Source: CAD feature listing. Evaluate the final solid. Frame: model axes, mm. Face numbers are marked on the shaded views. A direction names the side the tool comes from. Give positions to 0.01 mm unless a question says otherwise; leave off trailing zeros. Order: outer loops, then holes, each group sorted by start corner. A loop starts at its lowest first (then second) coordinate and runs counter-clockwise, first axis right, second up.
from build123d import *

# Parameters (mm, degrees)
SKETCH1_R           = 1.5
BOSS_EXTRUDE1_DEPTH = 1.5


with BuildPart() as part:
    # Sketch1 → Boss-Extrude1 (new body, symmetric)
    with BuildSketch(Plane.XY):
        with BuildLine():
            Line((-10.75, 18.625), (10.75, 18.625))
            ThreePointArc((10.75, 18.625), (14.25, 15.125), (10.75, 11.625))
            ThreePointArc((10.75, 11.625), (8.275126266, 10.599873734), (7.25, 8.125))
            Line((7.25, 8.125), (7.25, -8.125))
            ThreePointArc((7.25, -8.125), (8.275126266, -10.599873734), (10.75, -11.625))
            ThreePointArc((10.75, -11.625), (14.25, -15.125), (10.75, -18.625))
            Line((10.75, -18.625), (-10.75, -18.625))
            ThreePointArc((-10.75, -18.625), (-14.25, -15.125), (-10.75, -11.625))
            ThreePointArc((-10.75, -11.625), (-8.275126266, -10.599873734), (-7.25, -8.125))
            Line((-7.25, -8.125), (-7.25, 8.125))
            ThreePointArc((-7.25, 8.125), (-8.275126266, 10.599873734), (-10.75, 11.625))
            ThreePointArc((-10.75, 11.625), (-14.25, 15.125), (-10.75, 18.625))
        make_face()
        with Locations((-10.75, 15.125)):
            Circle(SKETCH1_R, mode=Mode.SUBTRACT)
        with Locations((10.75, 15.125)):
            Circle(SKETCH1_R, mode=Mode.SUBTRACT)
        with Locations((10.75, -15.125)):
            Circle(SKETCH1_R, mode=Mode.SUBTRACT)
        with Locations((-10.75, -15.125)):
            Circle(SKETCH1_R, mode=Mode.SUBTRACT)
    extrude(amount=BOSS_EXTRUDE1_DEPTH, both=True)


solid = part.part
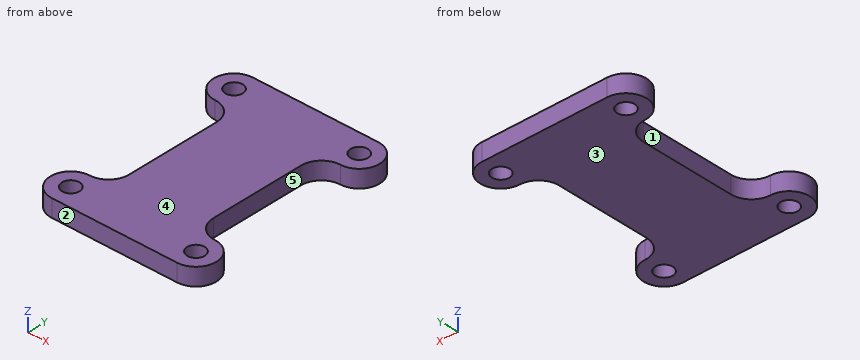
1) Reachability of the marked faces 4 and 5 from +Z, -Z, +X, -X, +Y, -Y: full face, straight path, thin tool, end or side. Return the list, or none.
Checks:
face 4: +Z, +X, -X, +Y, -Y
face 5: +Z, -Z, +X
2) First-contact query: pin 1 Ø2.5 at (x, y) = (-10.75, -15.125) entering from +Z; pin 2 Ø3.5 at (x, y) = (10.75, -15.125) entering from -Z. Flat tips, straight axial feed; report the tip coordinate or a pass-through.
Checks:
pin 1: passes through
pin 2: stops at z = -1.5
3) Section query A-A on z = -0.2. Output: boundary loops of the cut face in (x, y) (3 decimals), and give its area (3 significant figures).
Checks:
outline: (-10.75, -18.625) - (10.75, -18.625) arc R3.5 ccw to (10.75, -11.625) arc R3.5 cw to (7.25, -8.125) - (7.25, 8.125) arc R3.5 cw to (10.75, 11.625) arc R3.5 ccw to (10.75, 18.625) - (-10.75, 18.625) arc R3.5 ccw to (-10.75, 11.625) arc R3.5 cw to (-7.25, 8.125) - (-7.25, -8.125) arc R3.5 cw to (-10.75, -11.625) arc R3.5 ccw to start; hole circle Ø3 at (-10.75, -15.125); hole circle Ø3 at (-10.75, 15.125); hole circle Ø3 at (10.75, -15.125); hole circle Ø3 at (10.75, 15.125)
area: 697 mm2
4) Section query B-B on y = -16. Output: boundary loops of the cut face in (x, z), and give its area (3 significant figures).
Checks:
outline: (-14.14, -1.5) - (-11.97, -1.5) - (-11.97, 1.5) - (-14.14, 1.5) - close; (-9.53, -1.5) - (9.53, -1.5) - (9.53, 1.5) - (-9.53, 1.5) - close; (11.97, -1.5) - (14.14, -1.5) - (14.14, 1.5) - (11.97, 1.5) - close
area: 70.2 mm2
5) Section query D-D on y = 11. Output: boundary loops of the cut face in (x, z).
Checks:
outline: (-8.75, -1.5) - (8.75, -1.5) - (8.75, 1.5) - (-8.75, 1.5) - close
6) Pull-direction query (Y, two-part tool) for the marked faces 1, 2 and 3; classes: +Y half, -Y half, draft (parallel to the pull), parting line (faces both ways), or undercut.
Checks:
face 1: undercut
face 2: -Y half
face 3: draft
7) Ray query, L1, parallel to Y at x = 10.75, z = 0 (3 decimals); L2, parallel to X at y = -14.5, z = -1.25; L3, parallel to X at y = 7, z = 0. Return the intervals inside material, ascending.
Checks:
L1: y = -18.625 to -16.625, -13.625 to -11.625, 11.625 to 13.625, 16.625 to 18.625
L2: x = -14.19 to -12.11, -9.39 to 9.39, 12.11 to 14.19
L3: x = -7.25 to 7.25
8) Section query C-C on y = -2. Output: boundary loops of the cut face in (x, z).
Checks:
outline: (-7.25, -1.5) - (7.25, -1.5) - (7.25, 1.5) - (-7.25, 1.5) - close
